Autodesk Inventor part; units mm, degrees
ref_plane "YZ Plane" through (0, 0, 0) normal (1, 0, 0) x (0, 1, 0)
ref_plane "XZ Plane" through (0, 0, 0) normal (0, 1, 0) x (-1, 0, 0)
ref_plane "XY Plane" through (0, 0, 0) normal (0, 0, 1) x (1, 0, 0)
sketch "Sketch1" plane through (0, 0, 0) normal (0, 0, 1) x (1, 0, 0)
  line L0 (-29.415, -3) -> (12.585, -3)
  line L1 (12.585, -3) -> (12.585, -34)
  line L2 (12.585, -34) -> (-29.415, -34)
  line L3 (-29.415, -34) -> (-29.415, -3)
  line L4 (-29.6345, -34) -> (12.8045, -34)
  line L5 (-29.415, -3) -> (-15.931, -3)
  line L6 (-8.415, -407.2393) -> (-8.415, 249.8336) construction
  line L7 (-29.415, -18) -> (-29.415, -3) construction
  circle A0 centre (-21.915, -10.5) radius 2 construction
  circle A1 centre (5.085, -10.5) radius 2 construction
  circle A2 centre (-21.915, -29) radius 2.33 construction
  circle A3 centre (5.085, -29) radius 2.33 construction
  line L8 (-21.915, -10.5) -> (5.085, -10.5) construction
  line L9 (-21.915, -29) -> (5.085, -29) construction
  circle A4 centre (-21.915, -10.5) radius 2 construction
  circle A5 centre (5.085, -10.5) radius 2 construction
  circle A6 centre (5.085, -29) radius 2
  circle A7 centre (-21.915, -29) radius 2
  line L10 (-21.915, -10.5) -> (-21.915, -29) construction
  line L11 (-23.915, -10.5) -> (-23.915, -29)
  line L12 (-19.915, -29) -> (-19.915, -10.5)
  arc A8 (-19.915, -10.5) -> (-23.915, -10.5) centre (-21.915, -10.5) ccw
  arc A9 (-23.915, -29) -> (-19.915, -29) centre (-21.915, -29) ccw
  circle A10 centre (-21.915, -10.5) radius 2 construction
  line L13 (7.085, -10.5) -> (7.085, -29)
  line L14 (3.085, -29) -> (3.085, -10.5)
  arc A11 (7.085, -10.5) -> (3.085, -10.5) centre (5.085, -10.5) ccw
  arc A12 (3.085, -29) -> (7.085, -29) centre (5.085, -29) ccw
  point P0 (0, 0)
  point P1 (-8.415, -34)
  point P2 (-21.915, -19.75)
  point P3 (7.085, -29)
extrude "Plate1" add sketch "Sketch1" along normal blind 3
fillet "Fillet1" radius 2 4 edges at (-29.415, -34, 1.5) (12.585, -34, 1.5) (-29.415, -3, 1.5) (12.585, -3, 1.5)
equation "\"d7\" = Thickness"
equation "\"BendRadius\" = Thickness"
equation "\"BendReliefWidth\" = Thickness"
equation "\"BendReliefDepth\" = 0.5 * Thickness"
equation "\"CornerReliefSize\" = 4 * Thickness"
equation "\"MinimumRemnant\" = 2 * Thickness"
equation "\"TransitionRadius\" = BendRadius"
equation "\"JacobiRadiusSize\" = BendRadius"
equation "\"GapSize\" = Thickness"
properties part number "CameraMount"
The listing builds one solid part. Answer for the finished solid, in the listing's coordinates (mm). A direction names the side the tool comes from. Give positions to 0.01 mm unless a question says otherwise; leave off trailing zeros. Write each loop counter-clockwise with the first axis right and the second up, starting at its lowest first coordinate (ties: lowest second). Pieces come first, ordered by that corner, then holes. Notation, with made-up numbers: (35.25, 29) - (46.25, 29) arc R30 cw to (46.25, 64) - close; hole circle Ø11 at (76, -9.5). An arc over 180 degrees is marked (long way). Use a Markdown table: item, result.
1. A tool of negligible diameter and unlimited length cuts with its end or side. For faces 5 (the flat face through (-8, -34, 1)), 6 (the flat face through (-23.915, -20, 1)), from which of +Z, -Z, +X, -X, +Y, -Y can it reach the whole face along a straight path? Write none if from no direction.
Values follow:
| item | result |
|---|---|
| face 5 | +Z, -Z, +X, -X, -Y |
| face 6 | +Z, -Z |
2. For a pull along Y with two mould halves and no side action, classify faces 1 (the cylindrical face through (-28.845, -33.399, 1.521)), 2 (the cylindrical face through (5, -31, 1)), 3 (the flat face through (3.085, -20, 1)), 4 (the flat face through (-9, -18, 3)) as released by +Y, released by -Y, zero draft, split by the parting line, or undercut.
Values follow:
| item | result |
|---|---|
| face 1 | released by -Y |
| face 2 | undercut |
| face 3 | undercut |
| face 4 | zero draft |
3. Section B-B on z = 1.6 is taken. Write down the section's boundary in (x, y) (3 decimals).
Values follow:
| item | result |
|---|---|
| outline | (-29.415, -32) arc R2 ccw to (-27.415, -34) - (10.585, -34) arc R2 ccw to (12.585, -32) - (12.585, -5) arc R2 ccw to (10.585, -3) - (-27.415, -3) arc R2 ccw to (-29.415, -5) - close; hole (-23.915, -29) arc R2 ccw to (-19.915, -29) - (-19.915, -10.5) arc R2 ccw to (-23.915, -10.5) - close; hole (3.085, -29) arc R2 ccw to (7.085, -29) - (7.085, -10.5) arc R2 ccw to (3.085, -10.5) - close |
4. Find the intervals of material crossed by probe 1 along X at (y, z) = (-13, 0.45) (3 decimals); probe 2 along X at (y, z) = (-29.5, 1.7) (1 decimal); probe 3 along Y at (x, z) = (-20.5, 2.3), in increasing order. Write a range as from..to.
Values follow:
| item | result |
|---|---|
| probe 1 | x = -29.415..-23.915, -19.915..3.085, 7.085..12.585 |
| probe 2 | x = -29.4..-23.9, -20..3.1, 7..12.6 |
| probe 3 | y = -34..-30.41, -9.09..-3 |
5. Section A-A on y = -22 is taken. Write down the section's boundary in (x, z) (3 decimals).
Values follow:
| item | result |
|---|---|
| outline | (-29.415, 0) - (-23.915, 0) - (-23.915, 3) - (-29.415, 3) - close; (-19.915, 0) - (3.085, 0) - (3.085, 3) - (-19.915, 3) - close; (7.085, 0) - (12.585, 0) - (12.585, 3) - (7.085, 3) - close |
